For this review, take the finished solid that the model builds, in its own axes (mm). A direction names the side the tool comes from. Give positions to 0.01 mm unless a question says otherwise; leave off trailing zeros. Order: outer loops, then holes, each group sorted by start corner. A loop starts at its lowest first (then second) coordinate and runs counter-clockwise, first axis right, second up. Notation, with made-up numbers: (68.25, 47) - (98.25, 47) arc R31 cw to (98.25, 85) - close; hole circle Ø11 at (29, 75.5). An arc over 180 degrees is marked (long way). Use a Markdown table: item, result. Add a question column.
1) Machinability: for faces 4 (the face through (-20, -109, 17)), 5 (the face through (-69, -90, 18)), 6 (the face through (-86, -100, 14)), which of the approach directions +Z, -Z, +X, -X, +Y, -Y give a long, thin tool a straight path to every point of the face, cutting with its end or side? Answer none if there is none.
2) We need section C-C on x = -140. Write out the cut boundary in (y, z), then the cut area to 3 significant figures.
3) We need section B-B on y = -110. Write out the cut boundary in (x, z), then the cut area to 3 significant figures.
4) Clearance check with flat-ended pins moving along their axes: P1, Ø4, axis at x = -140, y = -30, coming from the -Z side; P2, Ø6.5, axis at x = -140, y = -80, coming from the -Z side; P3, Ø1.5, axis at x = -82.5, z = 18.5, coming from the +Y side; P4, Ø2.5, axis at y = -57.5, z = 18, coming from the +X side. State where each tip first meets the part, or that it passes through.
5) Wall thickness on L1, parallel to X at y = -110, z = 14; L2, parallel to Y at x = -140, z = 18.4; L3, parallel to Y at x = -105, z = 15.75: over which ranges is each line inside the solid? List them lowest first.
6) Mouldability with a two-part tool opening along X and no side actions: class faces 1 (the face through (-120, -55, 18)), 2 (the face through (-137.69, -79.04, 18.46)), 3 (the face through (-124, -72, 16)) as released by +X, released by -X, zero draft, split by the parting line, or undercut.
7) We need section D-D on z = 18.75. Write out the cut boundary in (x, y), then the cut area to 3 significant figures.
8) We need section A-A on y = -80. Write out the cut boundary in (x, z), then the cut area to 3 significant figures.
```python
from build123d import *

# Parameters (mm, degrees)
F1_DEPTH  = 12
F2_W      = 130
F2_H      = 20
F3_DEPTH  = 5
F4_W      = 105
F4_H      = 20
F5_DEPTH  = 5
F7_W      = 20
F7_H      = 100
F7_R      = 2.5
F7_H_2    = 20
F7_W_2    = 130
F8_DEPTH  = 25
F9_DEPTH  = 5
F10_W     = 130
F10_H     = 20
F10_W_2   = 20
F10_H_2   = 100
F11_DEPTH = 25
F12_W     = 100
F12_H     = 16
F13_DEPTH = 150
F14_W     = 80
F14_H     = 4
F15_DEPTH = 30.001


with BuildPart() as f1:
    # F0 (on Top) → F1 (new body)
    with BuildSketch(Plane.XY):
        with BuildLine():
            add(Edge.make_bspline(
                [(-116.5, 0), (-116.5, -86.5), (0, -86.5)],
                knots=[3.1415926536, 3.1415926536, 3.1415926536, 4.7123889804, 4.7123889804, 4.7123889804], degree=2, weights=[1, 0.7071067812, 1]))
            Line((-116.5, 0), (-116.5, -86.5))
            Line((-116.5, -86.5), (0, -86.5))
        make_face()
        Polygon((-116.5, -86.5), (-116.5, 0), (-130, 0), (-130, -100), (0, -100), (0, -86.5), align=None)
    extrude(amount=F1_DEPTH)

    # F2 (on face) → F3 (join)
    with BuildSketch(Plane.XZ.offset(100)):
        with Locations((-65, 6)):
            Rectangle(F2_W, F2_H)
    extrude(amount=F3_DEPTH)

    # F4 (on face) → F5 (join)
    with BuildSketch(Plane(origin=(-130, 0, 0), x_dir=(0, -1, 0), z_dir=(-1, 0, 0))):
        with Locations((52.5, 6)):
            Rectangle(F4_W, F4_H)
    extrude(amount=F5_DEPTH)

    # F7 (on face) → F8 (join)
    with BuildSketch(Plane(origin=(0, 0, -4), x_dir=(1, 0, 0), z_dir=(0, 0, -1))):
        with Locations((-140, 50)):
            Rectangle(F7_W, F7_H)
        with Locations((-140, 30)):
            Circle(F7_R, mode=Mode.SUBTRACT)
        with Locations((-140, 80)):
            Circle(F7_R, mode=Mode.SUBTRACT)
        with Locations((-140, 110)):
            Rectangle(F7_W, F7_H_2)
        with Locations((-65, 110)):
            Rectangle(F7_W_2, F7_H_2)
        with Locations((-105, 110)):
            Circle(F7_R, mode=Mode.SUBTRACT)
        with Locations((-30, 110)):
            Circle(F7_R, mode=Mode.SUBTRACT)
    extrude(amount=-F8_DEPTH)

    # F6 (on face) → F9 (join)
    with BuildSketch(Plane.XY.offset(16)):
        Polygon((-120, 0), (-135, 0), (-135, -105), (0, -105), (0, -90), (-120, -90), align=None)
    extrude(amount=F9_DEPTH)

    # F10 (on Top) → F11 (cut, symmetric)
    with BuildSketch(Plane.XY):
        with Locations((-85, -10)):
            Rectangle(F10_W, F10_H)
        with Locations((-10, -10)):
            Rectangle(F10_W_2, F10_H)
        with Locations((-10, -70)):
            Rectangle(F10_W_2, F10_H_2)
    extrude(amount=F11_DEPTH, both=True, mode=Mode.SUBTRACT)

    # F12 (on face) → F13 (cut)
    with BuildSketch(Plane.YZ.offset(-20)):
        with Locations((-70, 4)):
            Rectangle(F12_W, F12_H)
    extrude(amount=-F13_DEPTH, mode=Mode.SUBTRACT)

    # F14 (on face) → F15 (cut, through all)
    with BuildSketch(Plane.YZ.offset(-120)):
        with Locations((-60, 14)):
            Rectangle(F14_W, F14_H)
    extrude(amount=-F15_DEPTH, mode=Mode.SUBTRACT)


solid = f1.part
```
Checked values:
| question | item | result |
|---|---|---|
| 1 | face 4 | +Z, -Z, +X, +Y, -Y |
| 1 | face 5 | +Z, -Z, +X, +Y |
| 1 | face 6 | -Z, +X, -X, +Y |
| 2 | outline | (-120, 12) - (-100, 12) - (-100, 16) - (-82.5, 16) - (-82.5, 21) - (-120, 21) - close; (-77.5, 16) - (-32.5, 16) - (-32.5, 21) - (-77.5, 21) - close; (-27.5, 16) - (-20, 16) - (-20, 21) - (-27.5, 21) - close |
| 2 | area | 530 mm² |
| 3 | outline | (-150, 12) - (-107.5, 12) - (-107.5, 21) - (-150, 21) - close; (-102.5, 12) - (-32.5, 12) - (-32.5, 21) - (-102.5, 21) - close; (-27.5, 12) - (-20, 12) - (-20, 21) - (-27.5, 21) - close |
| 3 | area | 1,080 mm² |
| 4 | P1 | through |
| 4 | P2 | z = 16 |
| 4 | P3 | y = -90 |
| 4 | P4 | x = -120 |
| 5 | L1 | -150 to -107.5, -102.5 to -32.5, -27.5 to -20 |
| 5 | L2 | -120 to -82.5, -77.5 to -32.5, -27.5 to -20 |
| 5 | L3 | -120 to -112.5, -107.5 to -100 |
| 6 | face 1 | released by +X |
| 6 | face 2 | undercut |
| 6 | face 3 | zero draft |
| 7 | outline | (-150, -120) - (-20, -120) - (-20, -90) - (-120, -90) - (-120, -20) - (-150, -20) - close; hole circle Ø5 at (-140, -80); hole circle Ø5 at (-140, -30); hole circle Ø5 at (-105, -110); hole circle Ø5 at (-30, -110) |
| 7 | area | 5,920 mm² |
| 8 | outline | (-150, 16) - (-142.5, 16) - (-142.5, 21) - (-150, 21) - close; (-137.5, 16) - (-120, 16) - (-120, 21) - (-137.5, 21) - close |
| 8 | area | 125 mm² |
